Check sheet for the modelled part. Datum: model origin and axes. Units: mm. Face numbers are marked on the shaded views. A direction names the side the tool comes from. Round coordinates to 2 decimals unless told otherwise and drop trailing zeros. Order: outer loops, then holes, each group sorted by start corner. A loop starts at its lowest first (then second) coordinate and runs counter-clockwise, first axis right, second up. Notation, with made-up numbers: (-13.5, 84.25) -> (-2.5, 84.25) arc R14 cw to (-2.5, 88.25) -> close; hole circle Ø9 at (40, -19.5). An arc over 180 degrees is marked (long way). Answer in a Markdown table with one row per item.
from build123d import *

# Parameters (mm, degrees)
MAIN_BODY_R         = 37.34054
MAIN_BODY_R_2       = 30.99054
MAIN_BODY_R_3       = 26.03754
BOSS_EXTRUDE1_DEPTH = 57.15
MAIN_BODY_5_R       = 30.99054
MAIN_BODY_5_R_2     = 26.03754
CUT_EXTRUDE2_DEPTH  = 23.495
CUT_EXTRUDE3_START  = 31.877
MAIN_BODY_6_R       = 30.99054
MAIN_BODY_6_R_2     = 26.03754
CUT_EXTRUDE3_DEPTH  = 25.273
BOSS_EXTRUDE2_DEPTH = 21.59
BOSS_EXTRUDE3_DEPTH = 21.59


with BuildPart() as part:
    # Main Body → Boss-Extrude1 (new body)
    # profile 1 of 2: a face of its own
    with BuildSketch(Plane(origin=(0, -10.541, 0), x_dir=(-1, 0, 0), z_dir=(0, -1, 0))):
        with Locations(Location((0, 0, 0), (0, 0, 90))):
            Circle(MAIN_BODY_R)
        Circle(MAIN_BODY_R_2, mode=Mode.SUBTRACT)
    # profile 2 of 2: a face of its own
    with BuildSketch(Plane(origin=(0, -10.541, 0), x_dir=(-1, 0, 0), z_dir=(0, -1, 0))):
        Circle(MAIN_BODY_R_2)
        with Locations(Location((0, 0, 0), (0, 0, 90))):
            Circle(MAIN_BODY_R_3, mode=Mode.SUBTRACT)
    extrude(amount=BOSS_EXTRUDE1_DEPTH)

    # Main Body<5> → Cut-Extrude2 (cut)
    with BuildSketch(Plane(origin=(0, -10.541, 0), x_dir=(-1, 0, 0), z_dir=(0, -1, 0))):
        with Locations(Location((0, 0, 0), (0, 0, 90))):
            Circle(MAIN_BODY_5_R)
        with Locations(Location((0, 0, 0), (0, 0, 90))):
            Circle(MAIN_BODY_5_R_2, mode=Mode.SUBTRACT)
    extrude(amount=CUT_EXTRUDE2_DEPTH, mode=Mode.SUBTRACT)

    # Main Body<6> → Cut-Extrude3 (cut)
    with BuildSketch(Plane(origin=(0, -10.541, 0), x_dir=(-1, 0, 0), z_dir=(0, -1, 0)).offset(CUT_EXTRUDE3_START)):
        with Locations(Location((0, 0, 0), (0, 0, 90))):
            Circle(MAIN_BODY_6_R)
        with Locations(Location((0, 0, 0), (0, 0, 90))):
            Circle(MAIN_BODY_6_R_2, mode=Mode.SUBTRACT)
    extrude(amount=CUT_EXTRUDE3_DEPTH, mode=Mode.SUBTRACT)

    # Main Body<7> → Boss-Extrude2 (add)
    # profile 1 of 3: a face of its own
    with BuildSketch(Plane(origin=(0, -10.541, 0), x_dir=(-1, 0, 0), z_dir=(0, -1, 0))):
        with BuildLine():
            ThreePointArc((14.04286423, 34.599333689), (23.506970789, 33.71138504), (31.892042271, 38.188922533))
            Line((31.892042271, 38.188922533), (24.09649432, 88.732685748))
            Line((24.09649432, 88.732685748), (-30.227475734, 86.835650912))
            Line((-30.227475734, 86.835650912), (-34.657917418, 33.717474684))
            ThreePointArc((-34.657917418, 33.717474684), (-25.561615202, 31.465837631), (-16.422184031, 33.535470761))
            ThreePointArc((-16.422184031, 33.535470761), (-23.434260482, 34.041037689), (-26.454981852, 40.389270237))
            Line((-26.454981852, 40.389270237), (-25.562757718, 51.086469788))
            Line((-25.562757718, 51.086469788), (21.936876136, 52.745193552))
            Line((21.936876136, 52.745193552), (23.573125777, 42.136290252))
            ThreePointArc((23.573125777, 42.136290252), (21.002593049, 35.592806809), (14.04286423, 34.599333689))
        make_face()
        Polygon((17.597375259, 80.881086782), (20.76719935, 60.328992267), (-24.924949261, 58.733387277), (-23.196488344, 79.456533674), align=None, mode=Mode.SUBTRACT)
    # profile 2 of 3: a face of its own
    with BuildSketch(Plane(origin=(0, -10.541, 0), x_dir=(-1, 0, 0), z_dir=(0, -1, 0))):
        with BuildLine():
            ThreePointArc((14.04286423, 34.599333689), (29.288407022, 23.162580633), (36.904181225, 5.691865742))
            Line((36.904181225, 5.691865742), (31.892042271, 38.188922533))
            ThreePointArc((31.892042271, 38.188922533), (23.506970789, 33.71138504), (14.04286423, 34.599333689))
        make_face()
    # profile 3 of 3: a face of its own
    with BuildSketch(Plane(origin=(0, -10.541, 0), x_dir=(-1, 0, 0), z_dir=(0, -1, 0))):
        with BuildLine():
            ThreePointArc((-37.211328977, 3.103695095), (-30.832801883, 21.063101755), (-16.422184031, 33.535470761))
            ThreePointArc((-16.422184031, 33.535470761), (-25.561615202, 31.465837631), (-34.657917418, 33.717474684))
            Line((-34.657917418, 33.717474684), (-37.211328977, 3.103695095))
        make_face()
    extrude(amount=BOSS_EXTRUDE2_DEPTH)

    # Main Body<8> → Boss-Extrude3 (add)
    with BuildSketch(Plane(origin=(0, -10.541, 0), x_dir=(-1, 0, 0), z_dir=(0, -1, 0))):
        with BuildLine():
            ThreePointArc((37.099808191, -4.233220956), (30.17838959, -21.990469055), (15.395357729, -34.01909593))
            ThreePointArc((15.395357729, -34.01909593), (22.38882917, -34.737546541), (25.215213948, -41.174654833))
            Line((25.215213948, -41.174654833), (22.643322984, -63.714622021))
            Line((22.643322984, -63.714622021), (-18.14365763, -65.138934769))
            Line((-18.14365763, -65.138934769), (-22.281592226, -42.833279853))
            ThreePointArc((-22.281592226, -42.833279853), (-19.911122354, -36.214693398), (-12.984803239, -35.010152989))
            ThreePointArc((-12.984803239, -35.010152989), (-28.570898972, -24.042039419), (-36.714140357, -6.810860839))
            Line((-36.714140357, -6.810860839), (-16.240572134, -117.174216531))
            Line((-16.240572134, -117.174216531), (24.374671076, -115.755900985))
            Line((24.374671076, -115.755900985), (37.099808191, -4.233220956))
        make_face()
    extrude(amount=BOSS_EXTRUDE3_DEPTH)


solid = part.part
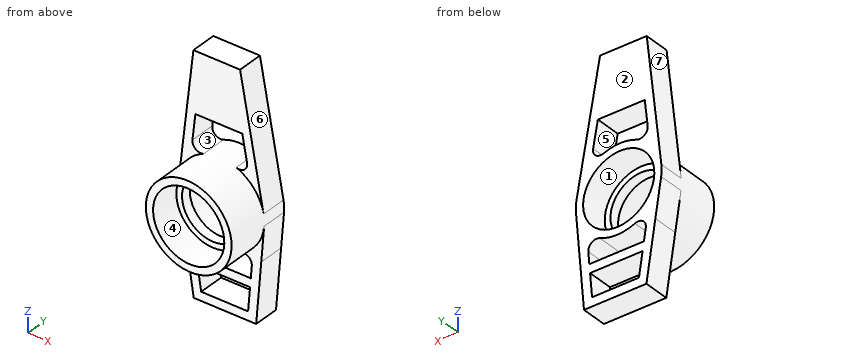
Item 1: Cross-section at A-A (z = -49). Record the boundary of the cut face in (x, y), and give its area (3 significant figures).
Result sheet:
| item | result |
|---|---|
| outline | (-30.22, -32.13) -> (-22.51, -32.13) -> (-22.51, -10.54) -> (-30.22, -10.54) -> close; (25.74, -32.13) -> (33.38, -32.13) -> (33.38, -10.54) -> (25.74, -10.54) -> close |
| area | 332 mm^2 |
Item 2: Cross-section at C-C (y = -28). Record the boundary of the cut face in (x, z) (1 decimal).
Result sheet:
| item | result |
|---|---|
| outline | (-37.1, 4.2) arc R37.3 ccw to (-36.9, -5.7) -> (-24.1, -88.7) -> (30.2, -86.8) -> (37.2, -3.1) arc R37.3 ccw to (36.7, 6.8) -> (16.2, 117.2) -> (-24.4, 115.8) -> close; hole circle Ø62 at (0, 0); hole (-25.2, 41.2) arc R7 ccw to (-15.4, 34) arc R37.3 cw to (13, 35) arc R7 ccw to (22.3, 42.8) -> (18.1, 65.1) -> (-22.6, 63.7) -> close; hole (-23.6, -42.1) -> (-21.9, -52.7) -> (25.6, -51.1) -> (26.5, -40.4) arc R7 ccw to (16.4, -33.5) arc R37.3 cw to (-14, -34.6) arc R7 ccw to start; hole (-20.8, -60.3) -> (-17.6, -80.9) -> (23.2, -79.5) -> (24.9, -58.7) -> close |
Item 3: Cross-section at B-B (x = 3.5). Record the boundary of the cut face in (y, z), and give its area (3 significant figures).
Result sheet:
| item | result |
|---|---|
| outline | (-67.69, -37.18) -> (-10.54, -37.18) -> (-10.54, -30.79) -> (-34.04, -30.79) -> (-34.04, -25.8) -> (-42.42, -25.8) -> (-42.42, -30.79) -> (-67.69, -30.79) -> close; (-67.69, 30.79) -> (-42.42, 30.79) -> (-42.42, 25.8) -> (-34.04, 25.8) -> (-34.04, 30.79) -> (-10.54, 30.79) -> (-10.54, 37.18) -> (-67.69, 37.18) -> close; (-32.13, -87.77) -> (-10.54, -87.77) -> (-10.54, -80.14) -> (-32.13, -80.14) -> close; (-32.13, -59.48) -> (-10.54, -59.48) -> (-10.54, -51.86) -> (-32.13, -51.86) -> close; (-32.13, 64.63) -> (-10.54, 64.63) -> (-10.54, 116.73) -> (-32.13, 116.73) -> close |
| area | 2,270 mm^2 |
Item 4: Set-up check for the marked faces 1, 2, 3 and 4: record each of +Z, -Z, +X, -X, +Y, -Y from which the full face is reachable in a straight line by a thin tool's end or side.
Result sheet:
| item | result |
|---|---|
| face 1 | +Y |
| face 2 | +Z, -Z, +X, -X, +Y |
| face 3 | +Y, -Y |
| face 4 | -Y |
Item 5: Cross-section at D-D (y = -51.5). Record the boundary of the cut face in (x, z).
Result sheet:
| item | result |
|---|---|
| outline | circle Ø74.68 at (0, 0); hole circle Ø61.98 at (0, 0) |
Item 6: Depth check by flat-ended pin: P1, Ø2, axis at y = -22, z = 85, coming from the +X side; P2, Ø1.5, axis at x = 16, y = -53, coming from the +Z side; P3, Ø1.5, axis at y = -30.5, z = 56.5, coming from the -X side; P4, Ø1, axis at x = 23.5, z = -36.5, coming from the -Y side. Enter the tip coordinate at first touch or a pass-through.
Result sheet:
| item | result |
|---|---|
| P1 | stops at x = 22.39 |
| P2 | stops at z = 34.08 |
| P3 | stops at x = -31.22 |
| P4 | passes through |
Item 7: Scan lines: line 1 (X direction, y = -40, z = 0); line 2 (Z direction, x = -3, y = -23) (3 decimals); line 3 (X direction, y = -48, z = 0). Record each from-to range of solid material in increasing order. Write a range as [from, to].
Result sheet:
| item | result |
|---|---|
| line 1 | x = [-37.34, -26.04], [26.04, 37.34] |
| line 2 | z = [-87.996, -80.371], [-59.709, -52.084], [-37.22, -30.845], [30.845, 37.22], [64.401, 116.502] |
| line 3 | x = [-37.34, -30.99], [30.99, 37.34] |
Item 8: Mould release check, pull along X, two halves, no side actions. Record for the marked faces 5, 6 and 7: pulls with the +X half, pulls with the -X half, needs draft (parallel to the pull), parting line crosses it, or undercut.
Result sheet:
| item | result |
|---|---|
| face 5 | undercut |
| face 6 | pulls with the +X half |
| face 7 | pulls with the -X half |
